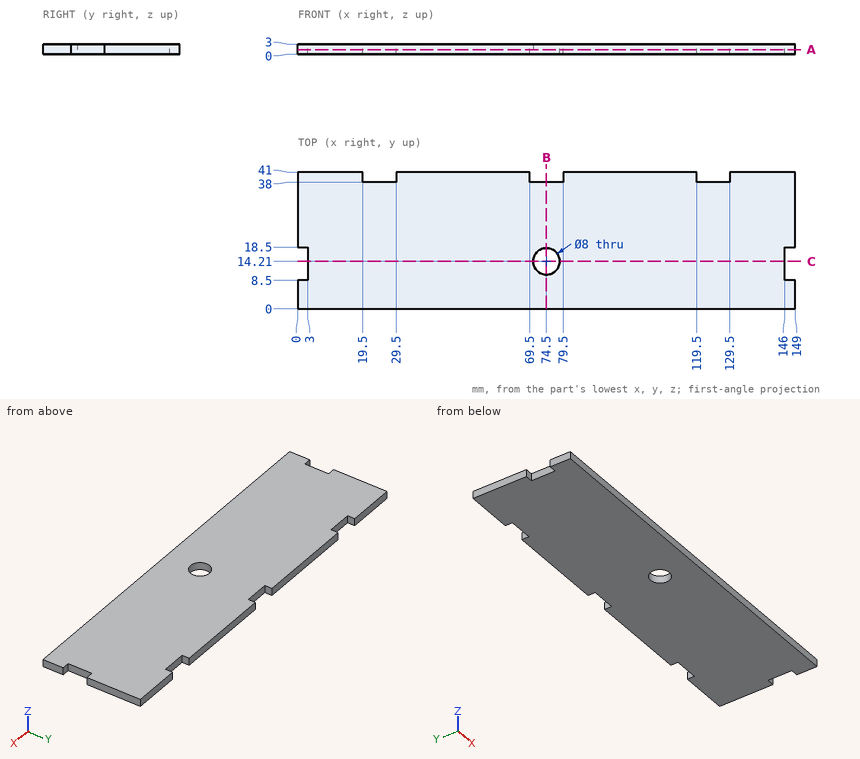
Here's the drawing with two shaded views (mm, measured from the low corner). I have some questions. Give positions to 0.01 mm unless a question says otherwise; leave off trailing zeros. Write each loop counter-clockwise with the first axis right and the second up, starting at its lowest first coordinate (ties: lowest second). Pieces come first, ordered by that corner, then holes. Notation, with made-up numbers: (30.5, 39.25) - (83.5, 39.25) arc R7 ccw to (83.5, 48.25) - close; hole circle Ø6 at (-18.75, 88). An arc over 180 degrees is marked (long way). Write item = value, one per line. Start each with the question number.
1. Imagine slicing it at A-A (z = 1.35). Please give me the cut outline in (x, y), and give its area (3 significant figures).
2. Imagine slicing it at B-B (x = 74.5). Please give me the cut outline in (y, z).
3. Imagine slicing it at C-C (y = 14.21). Please give me the cut outline in (x, z).
4. Please list where these lines run through material, in increasing order: line 1 (X direction, y = 39, z = 1.9); line 2 (X direction, y = 14.21, z = 1.8); line 3 (Y direction, x = 74.5, z = 2.05).
5. For pin 1 (0.9 mm diameter, centred on x = 22.5, z = 1.5, fed in from +Y), with a flat end and sliding along its axis, tell me the tip position at first contact or that it passes through.
Worked answers:
q1.outline = (0, 0) - (149, 0) - (149, 8.5) - (146, 8.5) - (146, 18.5) - (149, 18.5) - (149, 41) - (129.5, 41) - (129.5, 38) - (119.5, 38) - (119.5, 41) - (79.5, 41) - (79.5, 38) - (69.5, 38) - (69.5, 41) - (29.5, 41) - (29.5, 38) - (19.5, 38) - (19.5, 41) - (0, 41) - (0, 18.5) - (3, 18.5) - (3, 8.5) - (0, 8.5) - close; hole circle Ø8 at (74.5, 14.21)
q1.area = 5,910 mm2
q2.outline = (0, 0) - (10.21, 0) - (10.21, 3) - (0, 3) - close; (18.21, 0) - (38, 0) - (38, 3) - (18.21, 3) - close
q3.outline = (3, 0) - (70.5, 0) - (70.5, 3) - (3, 3) - close; (78.5, 0) - (146, 0) - (146, 3) - (78.5, 3) - close
q4.line_1 = 0 to 19.5, 29.5 to 69.5, 79.5 to 119.5, 129.5 to 149
q4.line_2 = 3 to 70.5, 78.5 to 146
q4.line_3 = 0 to 10.21, 18.21 to 38
q5.pin_1 = 38
